from build123d import *

# Parameters (mm, degrees)
SKETCH1_W           = 129.5
SKETCH1_H           = 36
BOSS_EXTRUDE1_DEPTH = 3
SKETCH2_W           = 50
SKETCH2_H           = 43
SKETCH2_R           = 2.25
BOSS_EXTRUDE2_DEPTH = 3


with BuildPart() as part:
    # Sketch1 → Boss-Extrude1 (new body)
    with BuildSketch(Plane(origin=(0, 0, 0), x_dir=(1, 0, 0), z_dir=(0, 1, 0))):
        with Locations((64.75, 18)):
            Rectangle(SKETCH1_W, SKETCH1_H)
    extrude(amount=BOSS_EXTRUDE1_DEPTH)

    # Sketch2 → Boss-Extrude2 (add)
    with BuildSketch(Plane(origin=(129.5, 0, 0), x_dir=(0, 0, -1), z_dir=(1, 0, 0))):
        with Locations((25, 21.5)):
            Rectangle(SKETCH2_W, SKETCH2_H)
        with Locations((40, 31)):
            Circle(SKETCH2_R, mode=Mode.SUBTRACT)
        with Locations((40, 13)):
            Circle(SKETCH2_R, mode=Mode.SUBTRACT)
    boss_extrude2 = extrude(amount=BOSS_EXTRUDE2_DEPTH)

    # Mirror1: Boss-Extrude2 across plane
    add(boss_extrude2.mirror(Plane(origin=(64.75, 0, 0), x_dir=(0, 0, 1), z_dir=(1, 0, 0))))


solid = part.part
Could you check a few things on this model? Use its own coordinates, in mm. A direction names the side the tool comes from. Coordinates: 2 decimals unless noted, no trailing zeros. Loops run counter-clockwise (first coordinate to the right, second up) from the corner with the lowest first, then second, coordinate; pieces in that order, holes last. Notation, with made-up numbers: (82.25, -14.75) -> (87.25, -14.75) arc R20 cw to (87.25, -4.75) -> close; hole circle Ø11 at (78.25, 48). An arc over 180 degrees is marked (long way). Answer in a Markdown table with one row per item.
(1) If I drill on probe 1 along Y at (x, z) = (-0.95, -40); probe 2 along X at (y, z) = (31, -6.5); probe 3 along Y at (x, z) = (27.5, -6.5), over which ranges is the centre line in solid material (lowest first)?
Results found:
| item | result |
|---|---|
| probe 1 | y = 0 to 10.75, 15.25 to 28.75, 33.25 to 43 |
| probe 2 | x = -3 to 0, 129.5 to 132.5 |
| probe 3 | y = 0 to 3 |
(2) For faces 4 (the face through (-1.479, 31.099, -37.752)), 5 (the face through (64, 1, -36)), 6 (the face through (64, 3, -18)), which set-ups out of +Z, -Z, +X, -X, +Y, -Y let a thin tool reach every point of the face, with its end or its side?
Results found:
| item | result |
|---|---|
| face 4 | +X, -X |
| face 5 | -Z, +Y, -Y |
| face 6 | +Z, -Z, +Y |
(3) Imagine slicing it at D-D (z = -8.5). List the corners of the cut face in (x, y) for me.
Results found:
| item | result |
|---|---|
| outline | (-3, 0) -> (132.5, 0) -> (132.5, 43) -> (129.5, 43) -> (129.5, 3) -> (0, 3) -> (0, 43) -> (-3, 43) -> close |
(4) Imagine slicing it at A-A (z = -40). List the corners of the cut face in (x, y) for me, plus the area to 3 significant figures.
Results found:
| item | result |
|---|---|
| outline | (-3, 0) -> (0, 0) -> (0, 10.75) -> (-3, 10.75) -> close; (-3, 15.25) -> (0, 15.25) -> (0, 28.75) -> (-3, 28.75) -> close; (-3, 33.25) -> (0, 33.25) -> (0, 43) -> (-3, 43) -> close; (129.5, 0) -> (132.5, 0) -> (132.5, 10.75) -> (129.5, 10.75) -> close; (129.5, 15.25) -> (132.5, 15.25) -> (132.5, 28.75) -> (129.5, 28.75) -> close; (129.5, 33.25) -> (132.5, 33.25) -> (132.5, 43) -> (129.5, 43) -> close |
| area | 204 mm^2 |
(5) Imagine slicing it at B-B (y = 13). List the corners of the cut face in (x, z) for me.
Results found:
| item | result |
|---|---|
| outline | (-3, -50) -> (0, -50) -> (0, -42.25) -> (-3, -42.25) -> close; (-3, -37.75) -> (0, -37.75) -> (0, 0) -> (-3, 0) -> close; (129.5, -50) -> (132.5, -50) -> (132.5, -42.25) -> (129.5, -42.25) -> close; (129.5, -37.75) -> (132.5, -37.75) -> (132.5, 0) -> (129.5, 0) -> close |
(6) Will these pins go through, and if not, where does the flat tip stop? pin 1 Ø10 at (x, z) = (15, -35) entering from +Y; pin 2 Ø1.5 at (x, y) = (42.5, 2) entering from -Z.
Results found:
| item | result |
|---|---|
| pin 1 | stops at y = 3 |
| pin 2 | stops at z = -36 |
(7) Thinking about a two-plate mould opening in X: for faces 1 (the face through (131, 43, -25)), 2 (the face through (-3, 22, -25)), 3 (the face through (129.5, 22, -25)), which applies, released by +X, released by -X, zero draft, split by the parting line, or undercut?
Results found:
| item | result |
|---|---|
| face 1 | zero draft |
| face 2 | released by -X |
| face 3 | undercut |
(8) Imagine slicing it at C-C (y = 19). List the corners of the cut face in (x, z) for me.
Results found:
| item | result |
|---|---|
| outline | (-3, -50) -> (0, -50) -> (0, 0) -> (-3, 0) -> close; (129.5, -50) -> (132.5, -50) -> (132.5, 0) -> (129.5, 0) -> close |
